Part model, mm, in its own coordinate system. Face numbers are marked on the shaded views. A direction names the side the tool comes from. Coordinates: 2 decimals unless noted, no trailing zeros. Write each loop counter-clockwise with the first axis right and the second up, starting at its lowest first coordinate (ties: lowest second). Pieces come first, ordered by that corner, then holes. Notation, with made-up numbers: (41, -13.75) -> (79, -13.75) arc R3 cw to (79, -8.75) -> close; hole circle Ø3 at (43, 54). An arc over 180 degrees is marked (long way). Write item = value, one per line.
from build123d import *

# Parameters (mm, degrees)
BOSS_EXTRUDE1_DEPTH = 20
SKETCH3_R           = 1.5
CUT_EXTRUDE2_DEPTH  = 77.182012842


with BuildPart() as part:
    # Sketch1 → Boss-Extrude1 (new body)
    with BuildSketch(Plane.XY):
        with BuildLine():
            Line((38.091006421, 10), (38.091006421, -10))
            ThreePointArc((38.091006421, -10), (0, -39.381782212), (-38.091006421, -10))
            Line((-38.091006421, -10), (-38.091006421, 10))
            ThreePointArc((-38.091006421, 10), (0, 39.381782212), (38.091006421, 10))
        make_face()
        with BuildLine():
            Line((-32.976154675, 10), (-32.976154675, -10))
            ThreePointArc((-32.976154675, -10), (0, -34.459059435), (32.976154675, -10))
            Line((32.976154675, -10), (32.976154675, 10))
            ThreePointArc((32.976154675, 10), (0, 34.459059435), (-32.976154675, 10))
        make_face(mode=Mode.SUBTRACT)
    extrude(amount=BOSS_EXTRUDE1_DEPTH)

    # Sketch3 → Cut-Extrude2 (cut, through all)
    with BuildSketch(Plane(origin=(38.091006421, 0, 0), x_dir=(0, 0, -1), z_dir=(1, 0, 0))):
        with Locations((-10, 5)):
            Circle(SKETCH3_R)
        with Locations((-10, -5)):
            Circle(SKETCH3_R)
    extrude(amount=-CUT_EXTRUDE2_DEPTH, mode=Mode.SUBTRACT)


solid = part.part
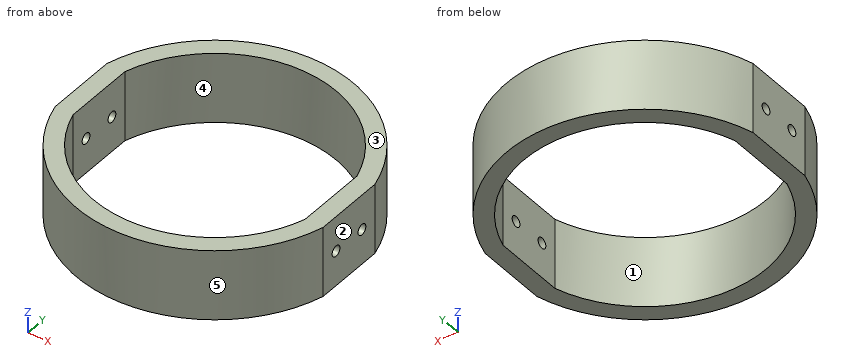
Q1. Probe line 1 (Y direction, x = 10, z = 16.25); line 2 (Y direction, x = 34.3, z = 10). List the from-to ranges inside material, lowest first. Write a range as from..to.
Model answer:
line_1 = -38.09..-32.98, 32.98..38.09
line_2 = -19.35..-6.5, -3.5..3.5, 6.5..19.35
Q2. Mould opens along X. For the marked faces 1, 2 and 3 say: released by +X, released by -X, zero draft, split by the parting line, or undercut.
Model answer:
face_1 = undercut
face_2 = released by +X
face_3 = zero draft
Q3. Saw through at A-A on y = -5. Give the cut face in (x, z), and give its area (3 significant figures).
Model answer:
outline = (-38.09, 0) -> (-32.98, 0) -> (-32.98, 8.5) -> (-38.09, 8.5) -> close; (-38.09, 11.5) -> (-32.98, 11.5) -> (-32.98, 20) -> (-38.09, 20) -> close; (32.98, 0) -> (38.09, 0) -> (38.09, 8.5) -> (32.98, 8.5) -> close; (32.98, 11.5) -> (38.09, 11.5) -> (38.09, 20) -> (32.98, 20) -> close
area = 174 mm²
Q4. Pin check, flat tips, straight feed: pin 1 (3.5 mm diameter, centred on y = -5, z = 10, fed in from +X); pin 2 (3 mm diameter, centred on x = -15, z = 9, fed in from -Y); pin 3 (3 mm diameter, centred on x = 22, z = 10.5, fed in from -Y); pin 4 (8 mm diameter, centred on x = 5, z = 5, fed in from -Y). Stop position of each tip, or through.
Model answer:
pin_1 = 38.09
pin_2 = -37
pin_3 = -33.63
pin_4 = -39.37
Q5. Saw through at B-B on x = 15.5. Give the cut face in (y, z).
Model answer:
outline = (-36.2, 0) -> (-30.78, 0) -> (-30.78, 20) -> (-36.2, 20) -> close; (30.78, 0) -> (36.2, 0) -> (36.2, 20) -> (30.78, 20) -> close
Q6. Saw through at D-D on y = 20. Give the cut face in (x, z), and give its area (3 significant figures).
Model answer:
outline = (-33.93, 0) -> (-28.06, 0) -> (-28.06, 20) -> (-33.93, 20) -> close; (28.06, 0) -> (33.93, 0) -> (33.93, 20) -> (28.06, 20) -> close
area = 235 mm²
Q7. Saw through at C-C on z = 16.5. Give the cut face in (x, y).
Model answer:
outline = (-38.09, -10) arc R39.38 ccw to (38.09, -10) -> (38.09, 10) arc R39.38 ccw to (-38.09, 10) -> close; hole (-32.98, -10) arc R34.46 ccw to (32.98, -10) -> (32.98, 10) arc R34.46 ccw to (-32.98, 10) -> close
Q8. Which spindle directions (+Z, -Z, +X, -X, +Y, -Y) get a long thin tool onto all of the face, cutting with end or side? Do the marked faces 4 and 5. Say none if no direction does.
Model answer:
face_4 = +Z, -Z
face_5 = +Z, -Z, -Y
